The listing builds one solid part. Answer for the finished solid, in the listing's coordinates (mm). Face numbers are marked on the shaded views. A direction names the side the tool comes from. Round coordinates to 2 decimals unless told otherwise and drop trailing zeros. Write each loop counter-clockwise with the first axis right and the second up, starting at its lowest first coordinate (ties: lowest second). Pieces come first, ordered by that corner, then holes.
from build123d import *

# Parameters (mm, degrees)
SKETCH3_W                                         = 133.096
SKETCH3_H                                         = 118.872
BOSS_EXTRUDE1_DEPTH                               = 50.8
BOSS_EXTRUDE2_DEPTH                               = 2.54
SKETCH11_W                                        = 121.92
SKETCH11_H                                        = 107.696
CUT_EXTRUDE1_DEPTH                                = 46.99
SKETCH12_W                                        = 16.456007839
SKETCH12_H                                        = 62.484
CUT_EXTRUDE2_DEPTH                                = 12.7
FILLET1_R                                         = 5.08
CSK_FOR_M2_5_FLAT_HEAD_MACHINE_SCREW1_D           = 2.9
CSK_FOR_M2_5_FLAT_HEAD_MACHINE_SCREW1_DEPTH       = 5.08
CSK_FOR_M2_5_FLAT_HEAD_MACHINE_SCREW1_CSINK_D     = 5.5
CSK_FOR_M2_5_FLAT_HEAD_MACHINE_SCREW1_CSINK_ANGLE = 90
CSK_FOR_M2_5_FLAT_HEAD_MACHINE_SCREW1_TIP         = 0.871247898


with BuildPart() as part:
    # Sketch3 → Boss-Extrude1 (new body)
    with BuildSketch(Plane.XY):
        with Locations((66.548, 59.436)):
            Rectangle(SKETCH3_W, SKETCH3_H)
    extrude(amount=BOSS_EXTRUDE1_DEPTH)

    # Sketch3<5> → Boss-Extrude2 (add)
    with BuildSketch(Plane.XY):
        Polygon((130.048, 115.824), (3.048, 115.824), (3.048, 74.168), (3.048, 11.684), (3.048, 3.048), (130.048, 3.048), align=None)
        Polygon((5.588, 74.168), (5.588, 113.284), (127.508, 113.284), (127.508, 5.588), (5.588, 5.588), (5.588, 11.684), align=None, mode=Mode.SUBTRACT)
    extrude(amount=-BOSS_EXTRUDE2_DEPTH)

    # Sketch11 → Cut-Extrude1 (cut)
    with BuildSketch(Plane(origin=(0, 0, 0), x_dir=(-1, 0, 0), z_dir=(0, 0, -1))):
        with Locations((-66.548, 59.436)):
            Rectangle(SKETCH11_W, SKETCH11_H)
    extrude(amount=-CUT_EXTRUDE1_DEPTH, mode=Mode.SUBTRACT)

    # Sketch12 → Cut-Extrude2 (cut)
    with BuildSketch(Plane.ZY):
        with Locations((5.688003919, 42.926)):
            Rectangle(SKETCH12_W, SKETCH12_H)
    extrude(amount=-CUT_EXTRUDE2_DEPTH, mode=Mode.SUBTRACT)

    # Fillet1
    fillet1_edges = [part.edges().sort_by_distance(p)[0] for p in [
        (133.096, 59.436, 50.8),
        (66.548, 118.872, 50.8),
        (0, 59.436, 50.8),
        (0, 118.872, 25.4),
        (133.096, 118.872, 25.4),
        (133.096, 0, 25.4),
        (0, 0, 25.4),
        (66.548, 0, 50.8),
    ]]
    fillet(fillet1_edges, radius=FILLET1_R)

    # CSK for M2.5 Flat Head Machine Screw1
    with Locations(Plane.XY.offset(50.8)):
        with Locations((12.7, 106.172), (120.396, 12.7)):
            CounterSinkHole(CSK_FOR_M2_5_FLAT_HEAD_MACHINE_SCREW1_D / 2, CSK_FOR_M2_5_FLAT_HEAD_MACHINE_SCREW1_CSINK_D / 2, depth=CSK_FOR_M2_5_FLAT_HEAD_MACHINE_SCREW1_DEPTH, counter_sink_angle=CSK_FOR_M2_5_FLAT_HEAD_MACHINE_SCREW1_CSINK_ANGLE)
            with Locations((0, 0, -(CSK_FOR_M2_5_FLAT_HEAD_MACHINE_SCREW1_DEPTH + CSK_FOR_M2_5_FLAT_HEAD_MACHINE_SCREW1_TIP / 2))):  # 118° drill point
                Cone(0, CSK_FOR_M2_5_FLAT_HEAD_MACHINE_SCREW1_D / 2, CSK_FOR_M2_5_FLAT_HEAD_MACHINE_SCREW1_TIP, mode=Mode.SUBTRACT)


solid = part.part
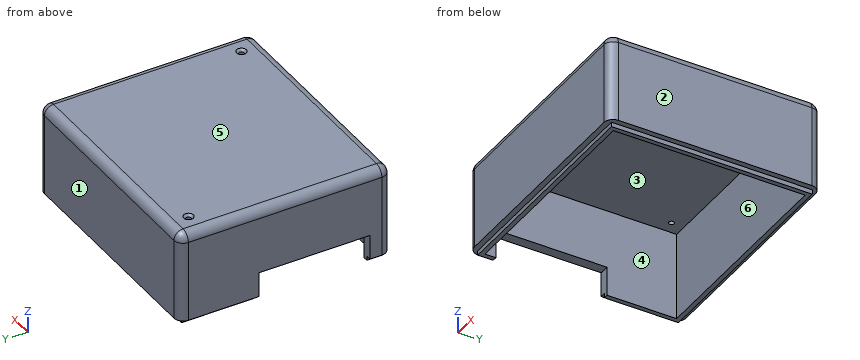
1. A tool of negligible diameter and unlimited length cuts with its end or side. For the marked faces 5 and 6, from which of +Z, -Z, +X, -X, +Y, -Y can it reach the whole face along a straight path? Write none if from no direction.
Geometry says:
face 5: +Z, +X, -X, +Y, -Y
face 6: -Z
2. For a pull along Y with two mould halves and no side action, classify the marked faces 1, 2, 3 and 4 as released by +Y, released by -Y, zero draft, split by the parting line, or undercut.
Geometry says:
face 1: released by +Y
face 2: zero draft
face 3: undercut
face 4: undercut
3. Section D-D on z = 1.5 is taken. Determine the outline of the cut face in (x, y).
Geometry says:
outline: (0, 5.08) arc R5.08 ccw to (5.08, 0) - (128.02, 0) arc R5.08 ccw to (133.1, 5.08) - (133.1, 113.79) arc R5.08 ccw to (128.02, 118.87) - (5.08, 118.87) arc R5.08 ccw to (0, 113.79) - (0, 74.17) - (5.59, 74.17) - (5.59, 113.28) - (127.51, 113.28) - (127.51, 5.59) - (5.59, 5.59) - (5.59, 11.68) - (0, 11.68) - close
4. Section C-C on x = 59 is taken. Determine the outline of the cut face in (y, z).
Geometry says:
outline: (0, 0) - (3.05, 0) - (3.05, -2.54) - (5.59, -2.54) - (5.59, 46.99) - (113.28, 46.99) - (113.28, -2.54) - (115.82, -2.54) - (115.82, 0) - (118.87, 0) - (118.87, 45.72) arc R5.08 ccw to (113.79, 50.8) - (5.08, 50.8) arc R5.08 ccw to (0, 45.72) - close
5. Section A-A on z = 33.5 is taken. Determine the outline of the cut face in (x, y).
Geometry says:
outline: (0, 5.08) arc R5.08 ccw to (5.08, 0) - (128.02, 0) arc R5.08 ccw to (133.1, 5.08) - (133.1, 113.79) arc R5.08 ccw to (128.02, 118.87) - (5.08, 118.87) arc R5.08 ccw to (0, 113.79) - close; hole (5.59, 5.59) - (127.51, 5.59) - (127.51, 113.28) - (5.59, 113.28) - close
6. Straight lines are drawn through the part: line 1 along X through (y, z) = (80, 24.5); line 2 along Y through (x, z) = (78, 35.5); line 3 along X through (y, z) = (24.5, 12). For each, find the intervals that lie inside material, in ascending order.
Geometry says:
line 1: x = 0 to 5.59, 127.51 to 133.1
line 2: y = 0 to 5.59, 113.28 to 118.87
line 3: x = 127.51 to 133.1
7. Section B-B on y = 67.5 is taken. Determine the outline of the cut face in (x, z).
Geometry says:
outline: (0, 13.92) - (5.59, 13.92) - (5.59, 46.99) - (127.51, 46.99) - (127.51, -2.54) - (130.05, -2.54) - (130.05, 0) - (133.1, 0) - (133.1, 45.72) arc R5.08 ccw to (128.02, 50.8) - (5.08, 50.8) arc R5.08 ccw to (0, 45.72) - close
8. Given pin 1 (4 mm diameter, centred on x = 33, y = 17.5, fed in from -Z); pin 2 (1.7 mm diameter, centred on x = 1.5, z = 3.5, fed in from +Y); pin 3 (1.7 mm diameter, centred on x = 120.396, y = 12.7, fed in from +Z); pin 4 (3 mm diameter, centred on x = 2.5, y = 51.5, fed in from -Z), each flat-ended and moving along its own axis, determine where each tip first touches the part or whether it passes through.
Geometry says:
pin 1: stops at z = 46.99
pin 2: stops at y = 118.08
pin 3: passes through
pin 4: stops at z = 13.92
